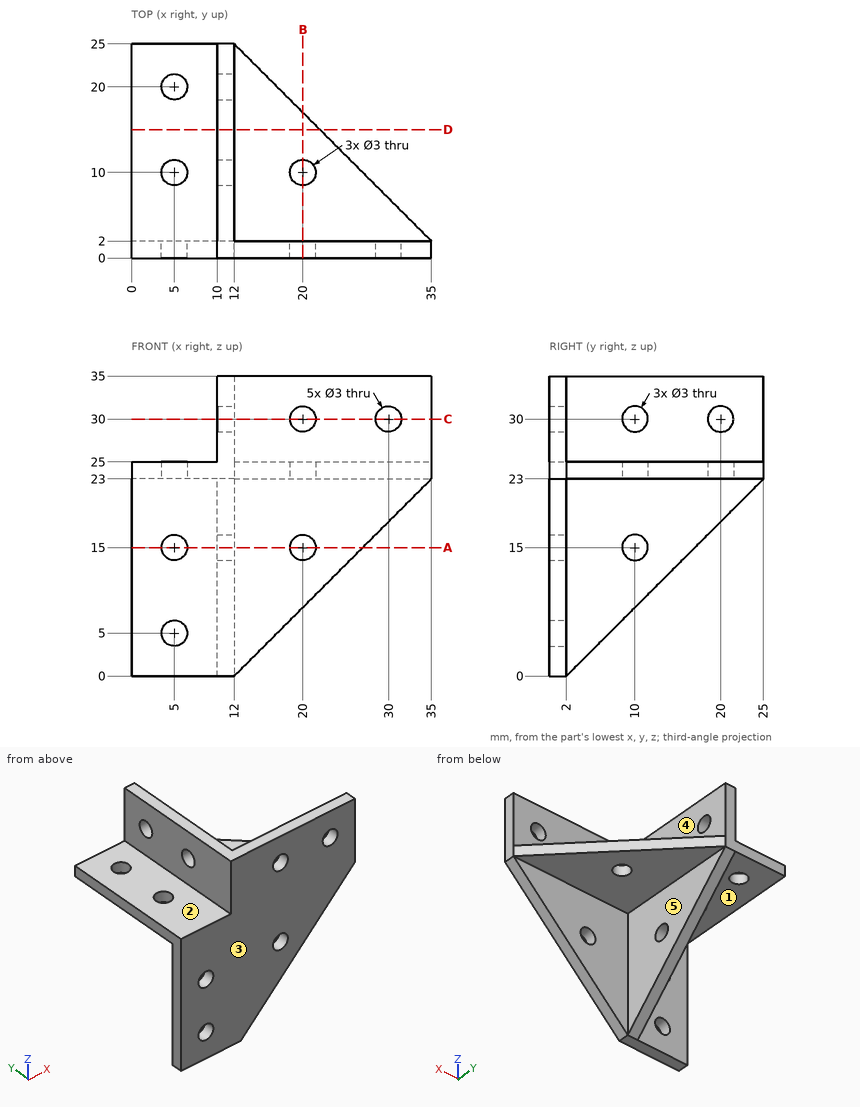
Print and shaded views of the part. All mm, measured from the part's lowest x, y and z. A direction names the side the tool comes from. Coordinates: 2 decimals unless noted, no trailing zeros. Order: outer loops, then holes, each group sorted by start corner. A loop starts at its lowest first (then second) coordinate and runs counter-clockwise, first axis right, second up. Notation, with made-up numbers: (-23, 64.25) -> (-7, 64.25) arc R8 ccw to (-7, 75.25) -> close; hole circle Ø5 at (62.25, 57.5). An arc over 180 degrees is marked (long way). Use one line per item in the form item = value. Start each with the question number.
1) Drop flat-ended pins along their axis: pin 1 (3 mm diameter, centred on y = 17.5, z = 32, fed in from -X); pin 2 (5 mm diameter, centred on y = 8, z = 7.5, fed in from +X); pin 3 (8 mm diameter, centred on x = 23, y = 6.5, fed in from -Z). Give the stop position or say it passes through.
2) Band-saw the part on A-A on z = 15. Give the cut face in (x, y), then the cut area to 3 significant figures.
3) Band-saw the part on B-B on x = 20. Give the cut face in (y, z).
4) Tool access for the marked faces 1, 2, 3, 4 and 5: list every direction of +Z, -Z, +X, -X, +Y, -Y with a clear straight run to the whole face (end or side of a thin tool).
5) Band-saw the part on D-D on y = 15. Give the cut face in (x, z), then the cut area to 3 significant figures.
6) Drill centre lines: L1, parallel to X at y = 1, z = 30; L2, parallel to Y at x = 10.5, z = 30; L3, parallel to X at y = 10, z = 23.8. Where is each one in solid material? Low to high. Write a range as [from, to].
7) Band-saw the part on C-C on z = 30. Give the cut face in (x, y).
Entries:
q1.pin_1 = 10
q1.pin_2 = 12
q1.pin_3 = 23
q2.outline = (0, 0) -> (3.5, 0) -> (3.5, 2) -> (0, 2) -> close; (6.5, 0) -> (18.5, 0) -> (18.5, 2) -> (12, 2) -> (12, 8.5) -> (10, 8.5) -> (10, 2) -> (6.5, 2) -> close; (10, 11.5) -> (12, 11.5) -> (12, 17) -> (10, 17) -> close; (21.5, 0) -> (27, 0) -> (27, 2) -> (21.5, 2) -> close
q2.area = 66.0 mm2
q3.outline = (0, 8) -> (2, 8) -> (2, 13.5) -> (0, 13.5) -> close; (0, 16.5) -> (2, 16.5) -> (2, 23) -> (8.5, 23) -> (8.5, 25) -> (2, 25) -> (2, 28.5) -> (0, 28.5) -> close; (0, 31.5) -> (2, 31.5) -> (2, 35) -> (0, 35) -> close; (11.5, 23) -> (17, 23) -> (17, 25) -> (11.5, 25) -> close
q4.face_1 = -Z, -X, +Y
q4.face_2 = +Z, -X, +Y, -Y
q4.face_3 = +Z, -Z, +X, -X, -Y
q4.face_4 = +Z, +X, +Y
q4.face_5 = -Z, +X, +Y
q5.outline = (0, 23) -> (10, 23) -> (10, 13) -> (12, 13) -> (12, 23) -> (22, 23) -> (22, 25) -> (12, 25) -> (12, 35) -> (10, 35) -> (10, 25) -> (0, 25) -> close
q5.area = 84.0 mm2
q6.L1 = [10, 18.5], [21.5, 28.5], [31.5, 35]
q6.L2 = [0, 8.5], [11.5, 18.5], [21.5, 25]
q6.L3 = [0, 3.5], [6.5, 18.5], [21.5, 27]
q7.outline = (10, 0) -> (18.5, 0) -> (18.5, 2) -> (12, 2) -> (12, 8.5) -> (10, 8.5) -> close; (10, 11.5) -> (12, 11.5) -> (12, 18.5) -> (10, 18.5) -> close; (10, 21.5) -> (12, 21.5) -> (12, 25) -> (10, 25) -> close; (21.5, 0) -> (28.5, 0) -> (28.5, 2) -> (21.5, 2) -> close; (31.5, 0) -> (35, 0) -> (35, 2) -> (31.5, 2) -> close
